Autodesk Inventor part; units mm, degrees
ref_plane "YZ Plane" through (0, 0, 0) normal (1, 0, 0) x (0, 1, 0)
ref_plane "XZ Plane" through (0, 0, 0) normal (0, 1, 0) x (-1, 0, 0)
ref_plane "XY Plane" through (0, 0, 0) normal (0, 0, 1) x (1, 0, 0)
sketch "Esboço1" plane through (0, 0, 0) normal (0, 0, 1) x (1, 0, 0)
  line L0 (66.9586, -53.8463) -> (66.9586, -18.5463)
  line L1 (66.9586, -18.5463) -> (46.3396, -18.5463)
  line L2 (46.3396, -18.5463) -> (46.3396, -53.8463)
  line L3 (46.3396, -53.8463) -> (66.9586, -53.8463)
  point P0 (0, 0)
  dimension "d0" = 35.3
  dimension "d1" = 20.619
extrude "Extrusão1" add sketch "Esboço1" along normal blind 2.5
chamfer "Chanfro1" distance 2.5 angle 45 2 edges at (56.6491, -18.5463, 0) (66.9586, -36.1963, 0)
sketch "Esboço2" plane through (0, 0, 2.5) normal (0, 0, 1) x (1, 0, 0)
  line L0 (66.9586, -18.5463) -> (46.3396, -18.5463)
  line L1 (46.3396, -18.5463) -> (46.3396, -11.6463)
  line L2 (46.3396, -11.6463) -> (66.9586, -11.6463)
  line L3 (66.9586, -11.6463) -> (66.9586, -18.5463)
  line L4 (66.9586, -18.5463) -> (46.3396, -18.5463)
  line L5 (46.3396, -18.5463) -> (46.3396, -19.5463)
  line L6 (46.3396, -19.5463) -> (66.9586, -19.5463)
  line L7 (66.9586, -19.5463) -> (66.9586, -18.5463)
  point P0 (0, 0)
  dimension "d7" = 6.9
  dimension "d10" = 1
extrude "Extrusão2" add sketch "Esboço2" along normal blind 2.5
chamfer "Chanfro2" distance 2.5 angle 45 1 edges at (56.6491, -19.5463, 2.5)
properties part number "suporte_placa"
Work out the finished part from the listing and answer in its coordinate system (mm). A direction names the side the tool comes from. Give positions to 0.01 mm unless a question says otherwise; leave off trailing zeros. Write each loop counter-clockwise with the first axis right and the second up, starting at its lowest first coordinate (ties: lowest second). Pieces come first, ordered by that corner, then holes. Notation, with made-up numbers: (-29, -21) -> (5, -21) arc R22 ccw to (5, -3) -> close; hole circle Ø5 at (58.25, 84.25). An arc over 180 degrees is marked (long way). Write each question's results on one line, items separated by ' | '.
1. Find section C-C on z = 4.6. Determine the outline of the cut face in (x, y).
Data:
outline: (46.34, -19.95) -> (66.96, -19.95) -> (66.96, -11.65) -> (46.34, -11.65) -> close
2. Each of these flat-tipped pins is pushed along its axis until it touches: pin 1 Ø2 at (x, y) = (51.5, -14.5) entering from -Z; pin 2 Ø8 at (x, y) = (60.5, -35.5) entering from +Z. Where does it stop, or does it pass through?
Data:
pin 1: z = 2.5 | pin 2: z = 2.5
3. A tool of negligible diameter and unlimited length cuts with its end or side. For faces 1 (the flat face through (57, -38, 2.5)), 2 (the flat face through (46.34, -32, 2)), 3 (the flat face through (57, -15, 2.5)), from which of +Z, -Z, +X, -X, +Y, -Y can it reach the whole face along a straight path? Write none if from no direction.
Data:
face 1: +Z, +X, -X, -Y | face 2: +Z, -Z, -X, +Y, -Y | face 3: -Z, +X, -X, +Y
4. Straight lines are drawn through the part: L1, parallel to Z at x = 47.5, y = -38; L2, parallel to Z at x = 60, y = -17.5; L3, parallel to Y at x = 58, z = 3.5. For each, find the intervals that lie inside material, in ascending order.
Data:
L1: 0 to 2.5 | L2: 2.5 to 5 | L3: -21.05 to -11.65
